Design review of the part built by this model. Coordinates are the model's own, in mm. Face numbers are marked on the shaded views. A direction names the side the tool comes from. Give positions to 0.01 mm unless a question says otherwise; leave off trailing zeros. Loops run counter-clockwise (first coordinate to the right, second up) from the corner with the lowest first, then second, coordinate; pieces in that order, holes last.
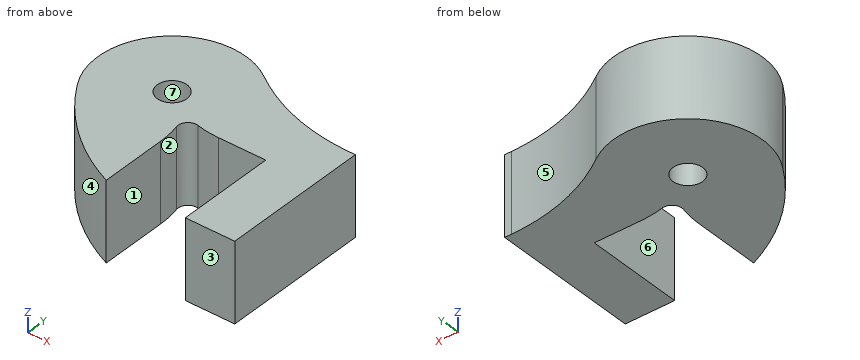
from build123d import *

# Parameters (mm, degrees)
SKETCH1_R           = 1.5
BOSS_EXTRUDE1_DEPTH = 8
SKETCH2_R           = 1
CUT_EXTRUDE1_DEPTH  = 27.248809497
FILLET1_R           = 10
BOSS_EXTRUDE2_DEPTH = 8
FILLET2_R           = 20
FILLET3_R           = 21


with BuildPart() as part:
    # Sketch1 → Boss-Extrude1 (new body)
    with BuildSketch(Plane.XY):
        Polygon((20, 0), (15, 0), (15, 10), (7, 10), (7, 0), (0, 0), (0, 15), (20, 15), align=None)
        with Locations((3.5, 12.5)):
            Circle(SKETCH1_R, mode=Mode.SUBTRACT)
    extrude(amount=BOSS_EXTRUDE1_DEPTH)

    # Sketch2 → Cut-Extrude1 (cut, through all)
    with BuildSketch(Plane.XY.offset(8)):
        with Locations((7.707106781, 9.292893219)):
            Circle(SKETCH2_R)
    extrude(amount=-CUT_EXTRUDE1_DEPTH, mode=Mode.SUBTRACT)

    # Fillet1
    fillet1_edges = [part.edges().sort_by_distance(p)[0] for p in [
        (8.414213562, 10, 4),
        (7, 8.585786438, 4),
    ]]
    fillet(fillet1_edges, radius=FILLET1_R)

    # Sketch3 → Boss-Extrude2 (add)
    with BuildSketch(Plane.XY.offset(8)):
        with BuildLine():
            Line((0, 15), (10.571067812, 15))
            ThreePointArc((10.571067812, 15), (-1.403283931, 18.175192217), (0, 5.866750419))
            Line((0, 5.866750419), (0, 15))
        make_face()
    extrude(amount=-BOSS_EXTRUDE2_DEPTH)

    # Fillet2
    # the kernel refuses this fillet: 20 mm, written as the material it adds along each edge
    with BuildSketch(Plane(origin=(10.571067812, 15, 8), x_dir=(1, 0, 0), z_dir=(0, 0, -1))) as fillet2_piece_1:
        with BuildLine():
            CenterArc((8.740320489, -20), FILLET2_R, 90, 35.096801228)
            Line((-2.758871003, -3.636363636), (-2.988854832, -3.309090909))
            ThreePointArc((-2.988854832, -3.309090909), (-1.414747274, -1.791391146), (-0.377123617, 0.133333333))
            Line((-0.377123617, 0.133333333), (0, 0.4))
            Line((0, 0.4), (8.740320489, 0.4))
            Line((8.740320489, 0.4), (8.740320489, 0))
        make_face()
    extrude(amount=8)
    with BuildSketch(Plane(origin=(0, 5.866750419, 8), x_dir=(0, -1, 0), z_dir=(0, 0, -1))) as fillet2_piece_2:
        with BuildLine():
            CenterArc((7.803057197, 19.906047223), FILLET2_R, 238.334677688, 26.109509541)
            Line((-2.696075005, 2.883467425), (-2.906057649, 2.543015829))
            ThreePointArc((-2.906057649, 2.543015829), (-1.447100359, 1.349108809), (-0.353773311, -0.186666667))
            Line((-0.353773311, -0.186666667), (0, -0.4))
            ThreePointArc((0, -0.4), (2.93337521, -0.4), (5.828024284, -0.398120944))
            Line((5.828024284, -0.398120944), (5.866750419, 0))
        make_face()
    extrude(amount=8)

    # Fillet3
    # the kernel refuses this fillet: 21 mm, written as the material it takes off along each edge
    with BuildSketch(Plane(origin=(0, 0, -22.27715114), x_dir=(-0.3161074470851615, 0.9487233958838066, 0), z_dir=(0, 0, 1))) as fillet3_piece_1:
        with BuildLine():
            CenterArc((13.589062195, -20.472284398), FILLET3_R, 102.871869537, 35.932692131)
            Line((-2.21275213, -6.641063771), (-2.528788416, -6.364439359))
            ThreePointArc((-2.528788416, -6.364439359), (-1.504839891, -3.187766758), (-0.398463826, 0.132765128))
            Line((-0.398463826, 0.132765128), (0.093564035, 0.409445688))
            ThreePointArc((0.093564035, 0.409445688), (4.455430228, -0.082586287), (8.817296421, 0.409445688))
            Line((8.817296421, 0.409445688), (8.910860456, 0))
        make_face()
    extrude(amount=52.55430228, mode=Mode.SUBTRACT)


solid = part.part
Q1. Insertion check: pin 1 (5 mm diameter, centred on x = 3.5, y = 12.5, fed in from -Z); pin 2 (3 mm diameter, centred on x = 4.5, z = 2, fed in from -Y); pin 3 (2 mm diameter, centred on y = 6, z = 4, fed in from -X); pin 4 (1 mm diameter, centred on x = 9.5, z = 4, fed in from -Y). Each pin has a flat end and moves straight along its axis. Give the tip position at first contact, or say it passes through.
Results:
pin 1: stops at z = 0
pin 2: stops at y = 0.45
pin 3: stops at x = -1.85
pin 4: stops at y = 10
Q2. Take a section at C-C (x = 3.5). Give the boundary of the cut face in (y, z).
Results:
outline: (1.88, 0) - (11, 0) - (11, 8) - (1.88, 8) - close; (14, 0) - (20, 0) - (20, 8) - (14, 8) - close
Q3. Take a section at B-B (z = 3). Give the boundary of the cut face in (x, y).
Results:
outline: (-2.88, 8.56) arc R20 cw to (-2.82, 8.45) arc R21 ccw to (7, 0) - (7, 6.77) arc R10 ccw to (6.73, 9.06) arc R1 cw to (7.94, 10.27) arc R10 ccw to (10.23, 10) - (15, 10) - (15, 0) - (20, 0) - (20, 15) - (19.31, 15) arc R20 cw to (7.81, 18.64) arc R7.5 ccw to start; hole circle Ø3 at (3.5, 12.5)
Q4. Take a section at D-D (x = 13.5). Give the boundary of the cut face in (y, z).
Results:
outline: (10, 0) - (15.86, 0) - (15.86, 8) - (10, 8) - close
Q5. Wall thickness on line 1 (Y direction, x = 3.5, z = 3.5); line 2 (Y direction, x = 4.75, z = 3); line 3 (X direction, y = 5.75, z = 1.5): over which ranges is each line inside the solid? List them lowest first.
Results:
line 1: y = 1.88 to 11, 14 to 20
line 2: y = 1.11 to 11.67, 13.33 to 19.9
line 3: x = -0.86 to 7, 15 to 20
Q6. Take a section at A-A (y = 12.5). Give the boundary of the cut face in (x, z).
Results:
outline: (-4, 0) - (2, 0) - (2, 8) - (-4, 8) - close; (5, 0) - (20, 0) - (20, 8) - (5, 8) - close
Q7. Tool access review of the marked faces 1, 2 and 3: name each direction out of +Z, -Z, +X, -X, +Y, -Y from which nothing blocks a thin tool from reaching the whole face with its end or side.
Results:
face 1: +Z, -Z, -Y
face 2: +Z, -Z
face 3: +Z, -Z, +X, -X, -Y
Q8. Draft analysis for pull direction Y (two halves, no side actions). For the marked faces 4, 5, 6 and 7, state which applies: pulls with the +Y half, pulls with the -Y half, needs draft (parallel to the pull), parting line crosses it, or undercut.
Results:
face 4: pulls with the -Y half
face 5: pulls with the +Y half
face 6: needs draft
face 7: undercut
